from build123d import *

# Parameters (mm, degrees)
SKETCH_1_R      = 4.5
EXTRUDE_1_DEPTH = 10


with BuildPart() as part:
    # Эскиз1 → Бобышка-Вытянуть1 (new body)
    with BuildSketch(Plane(origin=(0, 0, 0), x_dir=(1, 0, 0), z_dir=(0, 1, 0))):
        with BuildLine():
            Line((24.5, -7.5), (0, -7.5))
            ThreePointArc((0, -7.5), (-7.5, 0), (0, 7.5))
            Line((0, 7.5), (24.5, 7.5))
            Line((24.5, 7.5), (24.5, -7.5))
        make_face()
        with Locations(Location((0, 0, 0), (0, 0, 270))):
            Circle(SKETCH_1_R, mode=Mode.SUBTRACT)
    extrude(amount=EXTRUDE_1_DEPTH)


solid = part.part
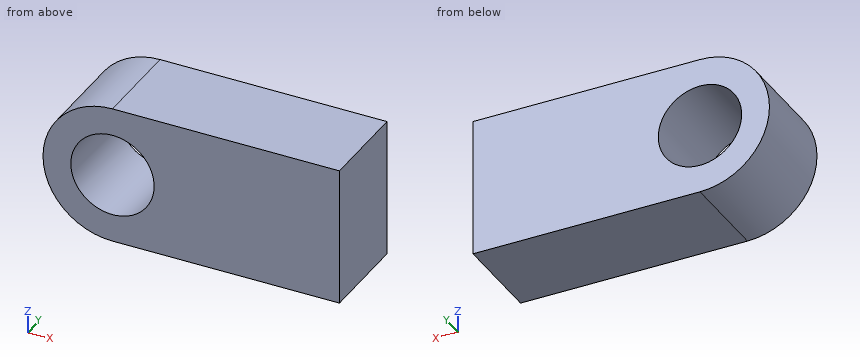
Work out the finished part from the listing and answer in its coordinate system (mm). Coordinates: 2 decimals unless noted, no trailing zeros. Write each loop counter-clockwise with the first axis right and the second up, starting at its lowest first coordinate (ties: lowest second). Pieces come first, ordered by that corner, then holes. Notation, with made-up numbers: M 22.25,10.5 L 46.25,10.5 A13 cw 46.25,15.5 Z; hole C -24.75,57.25 d8. An arc over 180 degrees is marked long. Answer as CSV lines item,"result". Start each with the question number.
Item 1: Section C-C on y = 2 is taken. Write down the section's boundary in (x, z), and give its area (3 significant figures).
Item 2: Flat-ended cylindrical pins translate along their axes: P1, Ø2, axis at x = 1, z = -3, coming from the +Y side; P2, Ø1, axis at y = 8.5, z = -4.5, coming from the -X side; P3, Ø1, axis at y = 6.5, z = 4, coming from the -X side; P4, Ø1, axis at y = 8.5, z = -3.5, coming from the -X side. Find the tip coordinate at first contact, or state that the pin passes through.
Item 3: Section B-B on x = -3 is taken. Write down the section's boundary in (y, z), and give its area (3 significant figures).
Item 4: Section A-A on z = 0 is taken. Write down the section's boundary in (x, y).
Item 5: Consider L1, parallel to X at y = 2, z = 0; L2, parallel to Z at x = -3.5, y = 7.5; L3, parallel to Z at x = -2, y = 1. Determine where each line is inside the solid, lowest interval first.
Checks:
1,outline,"M 0,-7.5 L 24.5,-7.5 L 24.5,7.5 L 0,7.5 A7.5 ccw Z; hole C 0,0 d9"
1,area,"392 mm²"
2,P1,"passes through"
2,P2,"stops at x = -6.34"
2,P3,"stops at x = -6.63"
2,P4,"stops at x = -6.87"
3,outline,"M 0,-6.87 L 10,-6.87 L 10,-3.35 L 0,-3.35 Z; M 0,3.35 L 10,3.35 L 10,6.87 L 0,6.87 Z"
3,area,"70.4 mm²"
4,outline,"M -7.5,0 L -4.5,0 L -4.5,10 L -7.5,10 Z; M 4.5,0 L 24.5,0 L 24.5,10 L 4.5,10 Z"
5,L1,"x = -7.5 to -4.5, 4.5 to 24.5"
5,L2,"z = -6.63 to -2.83, 2.83 to 6.63"
5,L3,"z = -7.23 to -4.03, 4.03 to 7.23"
